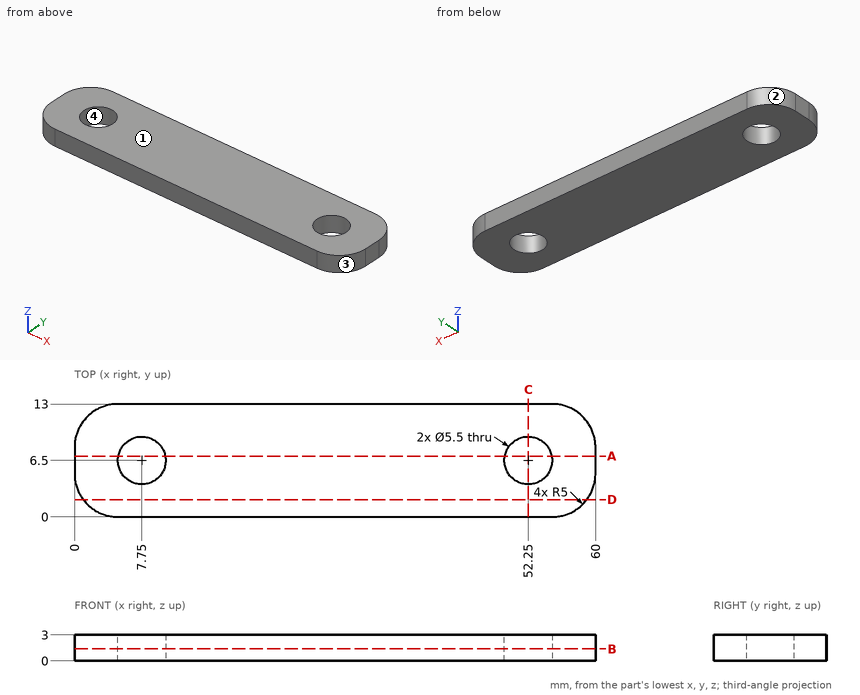
The figure shows three views and two pictorial views of one solid part (mm, origin at its lowest corner). Answer the questions. Give positions to 0.01 mm unless a question says otherwise; leave off trailing zeros. Write each loop counter-clockwise with the first axis right and the second up, starting at its lowest first coordinate (ties: lowest second). Pieces come first, ordered by that corner, then holes. Notation, with made-up numbers: (-19.5, 71.5) - (30.5, 71.5) arc R25 ccw to (30.5, 83.5) - close; hole circle Ø5 at (-35.75, 35). An arc over 180 degrees is marked (long way). Use one line per item in the form item = value. Start each with the question number.
1) Consider line 1 along Y through (x, z) = (7.75, 0.95); line 2 along X through (y, z) = (7.5, 1.9); line 3 along X through (y, z) = (4.75, 1.4). Determine where each line is inside the solid, lowest interval first. Write a range as from..to.
2) Find section D-D on y = 2. Determine the outline of the cut face in (x, z).
3) The mould has two halves that part along Y. Classify the marked faces 1, 2, 3 and 4: pulls with the +Y half, pulls with the -Y half, needs draft (parallel to the pull), parting line crosses it, or undercut.
4) Find section B-B on z = 1.4. Determine the outline of the cut face in (x, y), plus the area to 3 significant figures.
5) Find section A-A on y = 7. Determine the outline of the cut face in (x, z).
6) Find section C-C on x = 52.25. Determine the outline of the cut face in (y, z), plus the area to 3 significant figures.
Geometry results:
q1.line_1 = 0..3.75, 9.25..13
q1.line_2 = 0..5.19, 10.31..49.69, 54.81..60
q1.line_3 = 0.01..5.63, 9.87..50.13, 54.37..59.99
q2.outline = (1, 0) - (59, 0) - (59, 3) - (1, 3) - close
q3.face_1 = needs draft
q3.face_2 = pulls with the +Y half
q3.face_3 = pulls with the -Y half
q3.face_4 = undercut
q4.outline = (0, 5) arc R5 ccw to (5, 0) - (55, 0) arc R5 ccw to (60, 5) - (60, 8) arc R5 ccw to (55, 13) - (5, 13) arc R5 ccw to (0, 8) - close; hole circle Ø5.5 at (7.75, 6.5); hole circle Ø5.5 at (52.25, 6.5)
q4.area = 711 mm2
q5.outline = (0, 0) - (5.05, 0) - (5.05, 3) - (0, 3) - close; (10.45, 0) - (49.55, 0) - (49.55, 3) - (10.45, 3) - close; (54.95, 0) - (60, 0) - (60, 3) - (54.95, 3) - close
q6.outline = (0, 0) - (3.75, 0) - (3.75, 3) - (0, 3) - close; (9.25, 0) - (13, 0) - (13, 3) - (9.25, 3) - close
q6.area = 22.5 mm2
